Model file for the job. Use its own axes, mm. A direction names the side the tool comes from. Round coordinates to 2 decimals unless told otherwise and drop trailing zeros. Loops run counter-clockwise (first coordinate to the right, second up) from the corner with the lowest first, then second, coordinate; pieces in that order, holes last. Notation, with made-up numbers: M 7.25,63.25 L 29.25,63.25 A18 cw 29.25,94.25 Z; hole C -2,-38.75 d1. An arc over 180 degrees is marked long. Use a Markdown table: item, result. Add a question column.
Item 1: Saw through at C-C on y = 42. Write the cut outline in (x, z), then the cut area to 3 significant figures.
Item 2: Tool access for faces 5 (the flat face through (-27, 62, 79)), 6 (the flat face through (-1, 60, 73)), 7 (the flat face through (56, 42, 66)): list every direction of +Z, -Z, +X, -X, +Y, -Y with a clear straight run to the whole face (end or side of a thin tool).
Item 3: Two-plate mould, pull along Y, no slides. Class faces 1 (the cylindrical face through (-27.8, 62.06, 82.94)), 2 (the flat face through (-61, 48, 61)), 3 (the flat face through (59.62, 40.75, 63)), 4 (the cylindrical face through (25.2, 62.06, 82.94)): +Y half, -Y half, draft (parallel to the pull), parting line (faces both ways), or undercut.
Item 4: Saw through at A-A on x = -26.5. Write the cut outline in (y, z).
Item 5: Saw through at D-D on z = 84.5. Write the cut outline in (x, y).
Item 6: Saw through at B-B on y = 28. Write the cut outline in (x, z), then the cut area to 3 significant figures.
Item 7: Pin check, flat tips, straight feed: P1, Ø8, axis at y = 39, z = 84, coming from the -X side; P2, Ø2, axis at y = 39.5, z = 77.5, coming from the +X side; P3, Ø1.5, axis at x = -62, z = 61.5, coming from the +Y side. Stop position of each tip, or through.
Item 8: Wall check: L1, parallel to X at y = 22, z = 82.5; L2, parallel to Y at x = -26.5, z = 83.5; L3, parallel to X at y = 28.5, z = 74.25. Give the ranges that are in metal, low to high. Write a range as from..to.
```python
from build123d import *

# Parameters (mm, degrees)
SKETCH1_W        = 116
SKETCH1_H        = 44
SKETCH1_W_2      = 108
SKETCH1_H_2      = 36
WALLS_DEPTH      = 27
SKETCH2_W        = 6
SKETCH2_H        = 12
FLOOR_TABS_DEPTH = 3
SKETCH3_R        = 1.7
TAB_HOLES_DEPTH  = 5
SKETCH4_W        = 10
SKETCH4_H        = 4
BAR_BOSSES_DEPTH = 8
SKETCH5_R        = 1.3
BAR_PILOTS_DEPTH = 9
SKETCH6_W        = 22
SKETCH6_H        = 18
LEAD_EXIT_DEPTH  = 6


with BuildPart() as part:
    # Sketch1 → Walls (new body)
    with BuildSketch(Plane.XY.offset(60)):
        with Locations((0, 42)):
            Rectangle(SKETCH1_W, SKETCH1_H)
        with Locations((0, 42)):
            Rectangle(SKETCH1_W_2, SKETCH1_H_2, mode=Mode.SUBTRACT)
    extrude(amount=WALLS_DEPTH)

    # Sketch2 → Floor_tabs (add)
    with BuildSketch(Plane.XY.offset(60)):
        with Locations((61, 42)):
            Rectangle(SKETCH2_W, SKETCH2_H)
        with Locations((-61, 42)):
            Rectangle(SKETCH2_W, SKETCH2_H)
    extrude(amount=FLOOR_TABS_DEPTH)

    # Sketch3 → Tab_holes (cut)
    with BuildSketch(Plane.XY.offset(59)):
        with Locations((61, 42)):
            Circle(SKETCH3_R)
        with Locations((-61, 42)):
            Circle(SKETCH3_R)
    extrude(amount=TAB_HOLES_DEPTH, mode=Mode.SUBTRACT)

    # Sketch4 → Bar_bosses (add)
    with BuildSketch(Plane.XY.offset(79)):
        with Locations((26.5, 62)):
            Rectangle(SKETCH4_W, SKETCH4_H)
        with Locations((-26.5, 62)):
            Rectangle(SKETCH4_W, SKETCH4_H)
        with Locations((26.5, 22)):
            Rectangle(SKETCH4_W, SKETCH4_H)
        with Locations((-26.5, 22)):
            Rectangle(SKETCH4_W, SKETCH4_H)
    extrude(amount=BAR_BOSSES_DEPTH)

    # Sketch5 → Bar_pilots (cut)
    with BuildSketch(Plane.XY.offset(79)):
        with Locations((26.5, 62)):
            Circle(SKETCH5_R)
        with Locations((26.5, 22)):
            Circle(SKETCH5_R)
        with Locations((-26.5, 62)):
            Circle(SKETCH5_R)
        with Locations((-26.5, 22)):
            Circle(SKETCH5_R)
    extrude(amount=BAR_PILOTS_DEPTH, mode=Mode.SUBTRACT)

    # Sketch6 → Lead_exit (cut)
    with BuildSketch(Plane(origin=(53, 0, 0), x_dir=(0, 0, -1), z_dir=(1, 0, 0))):
        with Locations((-77, 42)):
            Rectangle(SKETCH6_W, SKETCH6_H)
    extrude(amount=LEAD_EXIT_DEPTH, mode=Mode.SUBTRACT)


solid = part.part
```
Entries:
| question | item | result |
|---|---|---|
| 1 | outline | M -64,60 L -62.7,60 L -62.7,63 L -64,63 Z; M -59.3,60 L -54,60 L -54,87 L -58,87 L -58,63 L -59.3,63 Z; M 54,60 L 59.3,60 L 59.3,63 L 58,63 L 58,66 L 54,66 Z; M 62.7,60 L 64,60 L 64,63 L 62.7,63 Z |
| 1 | area | 148 mm2 |
| 2 | face 5 | +Z |
| 2 | face 6 | +Z, -Z |
| 2 | face 7 | +Z, +X |
| 3 | face 1 | undercut |
| 3 | face 2 | +Y half |
| 3 | face 3 | draft |
| 3 | face 4 | undercut |
| 4 | outline | M 20,60 L 24,60 L 24,87 L 23.3,87 L 23.3,79 L 20.7,79 L 20.7,87 L 20,87 Z; M 60,60 L 64,60 L 64,87 L 63.3,87 L 63.3,79 L 60.7,79 L 60.7,87 L 60,87 Z |
| 5 | outline | M -58,20 L 58,20 L 58,33 L 54,33 L 54,24 L -54,24 L -54,60 L 54,60 L 54,51 L 58,51 L 58,64 L -58,64 Z; hole C -26.5,22 d2.6; hole C -26.5,62 d2.6; hole C 26.5,22 d2.6; hole C 26.5,62 d2.6 |
| 6 | outline | M -58,60 L -54,60 L -54,87 L -58,87 Z; M 54,60 L 58,60 L 58,87 L 54,87 Z |
| 6 | area | 216 mm2 |
| 7 | P1 | x = -58 |
| 7 | P2 | x = -54 |
| 7 | P3 | y = 48 |
| 8 | L1 | -58..-27.8, -25.2..25.2, 27.8..58 |
| 8 | L2 | 20..20.7, 23.3..24, 60..60.7, 63.3..64 |
| 8 | L3 | -58..-54, 54..58 |
